Design review of the part shown in the three views and the two pictorial views. Dimensions are in mm from the part's minimum x, y and z. A direction names the side the tool comes from. Coordinates: 2 decimals unless noted, no trailing zeros. Write each loop counter-clockwise with the first axis right and the second up, starting at its lowest first coordinate (ties: lowest second). Pieces come first, ordered by that corner, then holes. Notation, with made-up numbers: (-2, 83.25) -> (49, 83.25) arc R31 cw to (49, 110.25) -> close; hole circle Ø11 at (82, 62.25). An arc over 180 degrees is marked (long way). Write item = value, one per line. Start each with the question number.
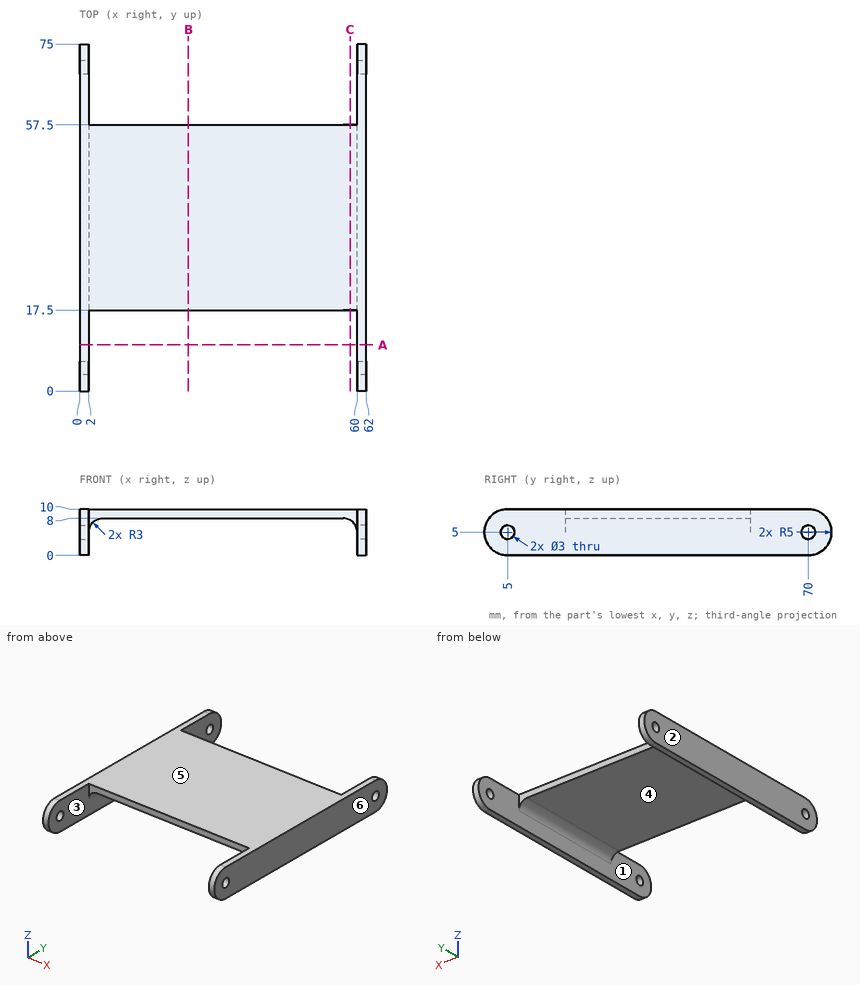
(1) For pin 1 Ø2.5 at (x, z) = (37.5, 6.5) entering from +Y; pin 2 Ø2 at (x, z) = (24, 7.5) entering from -Y; pin 3 Ø6 at (x, y) = (16, 59.5) entering from -Z, all flat-tipped, find the tip position at first contact; note any pin that passes through.
(2) For line 1 (X direction, y = 69, z = 8.75); line 2 (Z direction, x = 61, y = 70); line 3 (Z direction, x = 30, y = 23), list the stretches that pass through material, from the lowest coordinate up.
(3) Take a section at A-A, the plane y = 10. State the section outline as (x, z) points.
(4) Take a section at C-C, the plane x = 58.5. State the section outline as (y, z) points, then the cut area to 3 significant figures.
(5) For the marked faces 1 and 2, list the 3-axis set-ups (+Z, -Z, +X, -X, +Y, -Y) from which the entire face can be reached by the end or side of a thin tool; tool diameter is ignored.
(6) Mouldability with a two-part tool opening along X and no side actions: class the marked faces 3, 4, 5 and 6 as pulls with the +X half, pulls with the -X half, needs draft (parallel to the pull), parting line crosses it, or undercut.
(7) Take a section at B-B, the plane x = 23.5. State the section outline as (y, z) points.
Report:
q1.pin_1 = through
q1.pin_2 = 17.5
q1.pin_3 = 8
q2.line_1 = 0 to 2, 60 to 62
q2.line_2 = 0 to 3.5, 6.5 to 10
q2.line_3 = 8 to 10
q3.outline = (0, 0) -> (2, 0) -> (2, 10) -> (0, 10) -> close; (60, 0) -> (62, 0) -> (62, 10) -> (60, 10) -> close
q4.outline = (17.5, 7.6) -> (57.5, 7.6) -> (57.5, 10) -> (17.5, 10) -> close
q4.area = 96.1 mm2
q5.face_1 = -Z
q5.face_2 = +Z, -Z, -X, +Y, -Y
q6.face_3 = undercut
q6.face_4 = undercut
q6.face_5 = needs draft
q6.face_6 = pulls with the +X half
q7.outline = (17.5, 8) -> (57.5, 8) -> (57.5, 10) -> (17.5, 10) -> close
